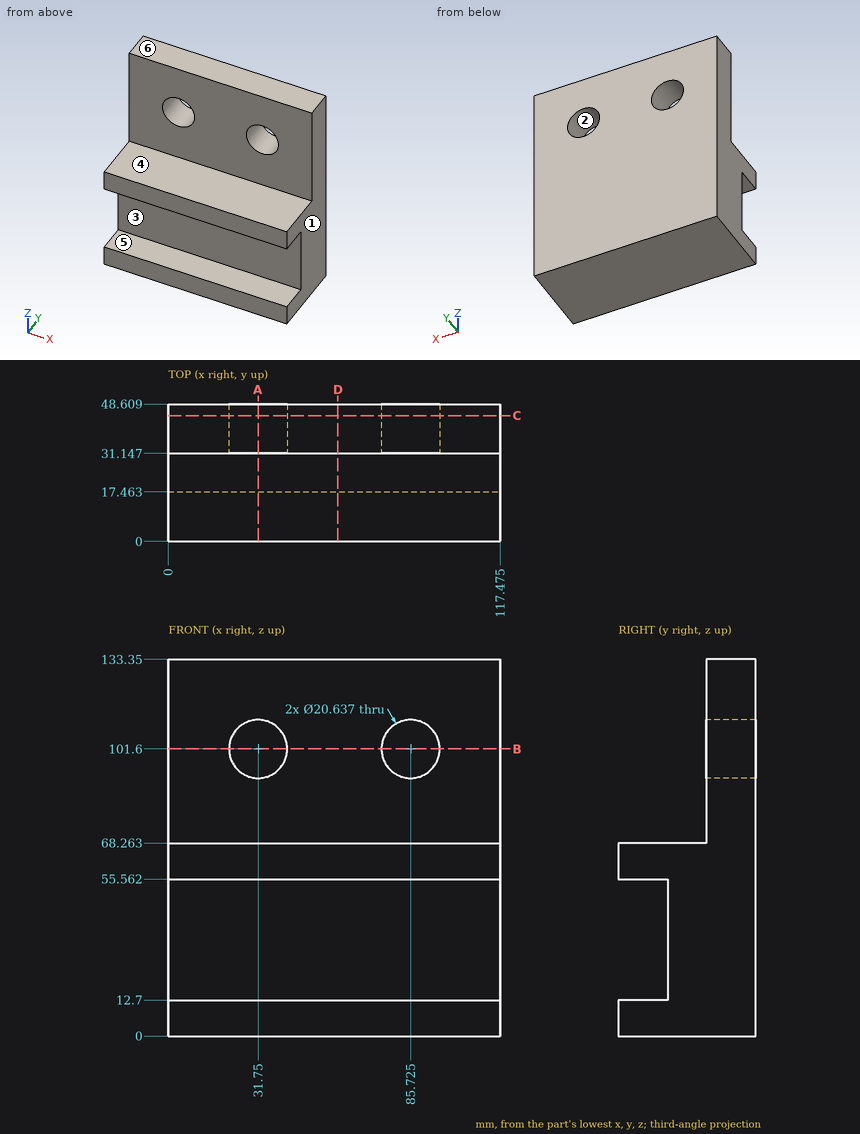
Geometry check sheet. Reference: drawing and pictorial views, mm from the part's lowest x, y, z. A direction names the side the tool comes from. Coordinates: 2 decimals unless noted, no trailing zeros. Loops run counter-clockwise (first coordinate to the right, second up) from the corner with the lowest first, then second, coordinate; pieces in that order, holes last. Notation, with made-up numbers: (61, 79) -> (101, 79) arc R23 ccw to (101, 103) -> close; hole circle Ø1 at (64, 5). An arc over 180 degrees is marked (long way). Write item = value, one per line. Start each with the question number.
1. Section check C-C on y = 44.5. Give the number of separate pieces and of enclosed holes in the cut face, then the cut area to 3 significant figures.
2. Tool access check on the marked faces 4, 5 and 6. Record the directions out of +Z, -Z, +X, -X, +Y, -Y that give a thin tool (end or side, any length) a straight path to the whole face; none if there is none.
3. Section check A-A on x = 31.75. Record the cut outline in (y, z).
4. Draft check along X on the marked faces 1, 2 and 3. Enter one of: released by +X, released by -X, zero draft, split by the parting line, or undercut.
5. Depth check by flat-ended pin: P1, Ø2, axis at x = 53, z = 108.5, coming from the -Y side; P2, Ø9.5, axis at x = 73, y = 22.5, coming from the +Z side; P3, Ø16.5, axis at x = 85.725, z = 101.6, coming from the -Y side. Enter the tip coordinate at first touch or a pass-through.
6. Section check D-D on x = 60. Record the cut outline in (y, z).
7. Section check B-B on z = 101.6. Record the cut outline in (x, y) (1 decimal), then the cut area to 3 significant figures.
8. Material ranges on line 1 (X direction, y = 39, z = 101) (1 decimal); line 2 (Z direction, x = 68, y = 9.5); line 3 (Y direction, x = 71, z = 111), recorded low to high.
Responses:
q1.separate_pieces = 1
q1.enclosed_holes = 2
q1.area = 15,000 mm2
q2.face_4 = +Z, +X, -X, -Y
q2.face_5 = +X, -X, -Y
q2.face_6 = +Z, +X, -X, +Y, -Y
q3.outline = (0, 0) -> (48.61, 0) -> (48.61, 91.28) -> (31.15, 91.28) -> (31.15, 68.26) -> (0, 68.26) -> (0, 55.56) -> (17.46, 55.56) -> (17.46, 12.7) -> (0, 12.7) -> close; (31.15, 111.92) -> (48.61, 111.92) -> (48.61, 133.35) -> (31.15, 133.35) -> close
q4.face_1 = released by +X
q4.face_2 = undercut
q4.face_3 = zero draft
q5.P1 = 31.15
q5.P2 = 68.26
q5.P3 = through
q6.outline = (0, 0) -> (48.61, 0) -> (48.61, 133.35) -> (31.15, 133.35) -> (31.15, 68.26) -> (0, 68.26) -> (0, 55.56) -> (17.46, 55.56) -> (17.46, 12.7) -> (0, 12.7) -> close
q7.outline = (0, 31.1) -> (21.4, 31.1) -> (21.4, 48.6) -> (0, 48.6) -> close; (42.1, 31.1) -> (75.4, 31.1) -> (75.4, 48.6) -> (42.1, 48.6) -> close; (96, 31.1) -> (117.5, 31.1) -> (117.5, 48.6) -> (96, 48.6) -> close
q7.area = 1,330 mm2
q8.line_1 = 0 to 21.4, 42.1 to 75.4, 96 to 117.5
q8.line_2 = 0 to 12.7, 55.56 to 68.26
q8.line_3 = 31.15 to 48.61
